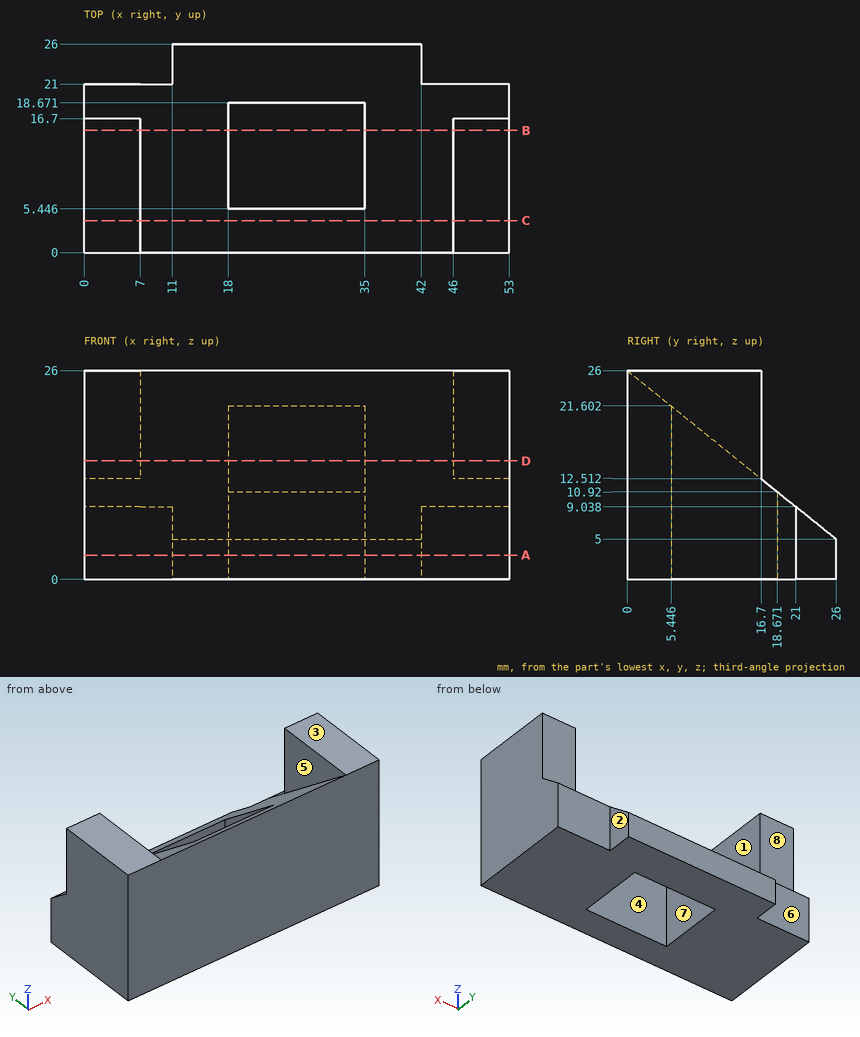
Answer from the drawing. Dimensions are ordinates in mm from the lowest x, y and z of the part. A direction names the side the tool comes from. Round coordinates to 2 decimals unless told otherwise and drop trailing zeros. Order: outer loops, then holes, each group sorted by start corner. A loop starts at its lowest first (then second) coordinate and runs counter-clockwise, first axis right, second up. Notation, with made-up numbers: (3.25, 49.25) - (47.25, 49.25) arc R15 cw to (47.25, 66.25) - close; hole circle Ø7 at (35, 4.5). An arc over 180 degrees is marked (long way). Put each result on its own line as item: value. Start each with the question number.
(1) Find section A-A (z = 3). Give the vertices of the cut face in (x, y) (1 decimal).
(2) Find section D-D (z = 14.75). Give the vertices of the cut face in (x, y) (1 decimal).
(3) For the marked faces 5, 6, 7 and 8, determine the directions among +Z, -Z, +X, -X, +Y, -Y from which every point of the face is accessible in a straight line to the end or side of a thin tool.
(4) Find section B-B (y = 15.25). Give the vertices of the cut face in (x, z), plus the area to 3 significant figures.
(5) Find section C-C (y = 4). Give the vertices of the cut face in (x, z).
(6) Straight lines are drawn through the part: probe 1 along X at (y, z) = (9.5, 3.75); probe 2 along X at (y, z) = (6.5, 21.25); probe 3 along Y at (x, z) = (31.5, 20.25) (1 decimal). For each, find the intervals that lie inside material, in ascending order. Write a range as from..to.
(7) Given P1, Ø5, axis at x = 27, y = 22.5, coming from the +Z side (1 decimal); P2, Ø2, axis at x = 50.5, z = 22, coming from the +Y side; P3, Ø4.5, axis at x = 46.5, z = 5.5, coming from the +Y side, each flat-ended and moving along its own axis, determine where each tip first touches the part or whether it passes through.
(8) Determine the mould class of the marked faces 1, 2, 3 and 4 for opening direction X: released by +X, released by -X, zero draft, split by the parting line, or undercut.
Reply:
1. outline: (0, 0) - (53, 0) - (53, 21) - (42, 21) - (42, 26) - (11, 26) - (11, 21) - (0, 21) - close; hole (18, 5.4) - (35, 5.4) - (35, 18.7) - (18, 18.7) - close
2. outline: (0, 0) - (53, 0) - (53, 16.7) - (46, 16.7) - (46, 13.9) - (35, 13.9) - (35, 5.4) - (18, 5.4) - (18, 13.9) - (7, 13.9) - (7, 16.7) - (0, 16.7) - close
3. face 5: +Z, +Y
3. face 6: +Z, -Z, -X, +Y
3. face 7: +Z, -Z
3. face 8: +Z, +X, -X, +Y
4. outline: (0, 0) - (18, 0) - (18, 13.68) - (7, 13.68) - (7, 26) - (0, 26) - close; (35, 0) - (53, 0) - (53, 26) - (46, 26) - (46, 13.68) - (35, 13.68) - close
4. area: 665 mm^2
5. outline: (0, 0) - (53, 0) - (53, 26) - (46, 26) - (46, 22.77) - (7, 22.77) - (7, 26) - (0, 26) - close
6. probe 1: 0..18, 35..53
6. probe 2: 0..7, 46..53
6. probe 3: 0..5.4
7. P1: z = 9.8
7. P2: y = 16.7
7. P3: y = 21
8. face 1: undercut
8. face 2: released by +X
8. face 3: zero draft
8. face 4: undercut
